Here's how the part is built. I have some questions about the finished solid (model axes, mm). Coordinates: 2 decimals unless noted, no trailing zeros. Loops run counter-clockwise (first coordinate to the right, second up) from the corner with the lowest first, then second, coordinate; pieces in that order, holes last. Notation, with made-up numbers: (-14, -27) -> (23, -27) arc R19 cw to (23, 5) -> close; hole circle Ø8 at (14, -26). An arc over 180 degrees is marked (long way). Answer as a JSON object with one key per item and string values. Group by question number.
1) I'm going to push flat-ended pins straight in: pin 1 (4.5 mm diameter, centred on x = 38.1, y = 88.9, fed in from +Z); pin 2 (1.6 mm diameter, centred on y = 47, z = 2, fed in from +X). Where does each tip first touch, or does it pass through?
2) I need wall thicknesses on probe 1 along Y at (x, z) = (38.1, 1.5); probe 2 along Y at (x, z) = (63.5, 1.9); probe 3 along Y at (x, z) = (40, 0.25). Which ranges of each line are inside material? Lowest first, please. Write a range as [from, to].
3) I want a section at D-D (x = 12.7). Write out the boundary of the cut face in (y, z) (3 decimals).
4) I want a section at B-B (y = 101.6). Write out the boundary of the cut face in (x, z) (3 decimals).
5) I want a section at A-A (x = 63.5). Write out the boundary of the cut face in (y, z) (3 decimals).
6) I want a section at C-C (z = 0.9). Count the separate pieces of the cut face and the enclosed holes in it, then the cut area to 3 significant figures.
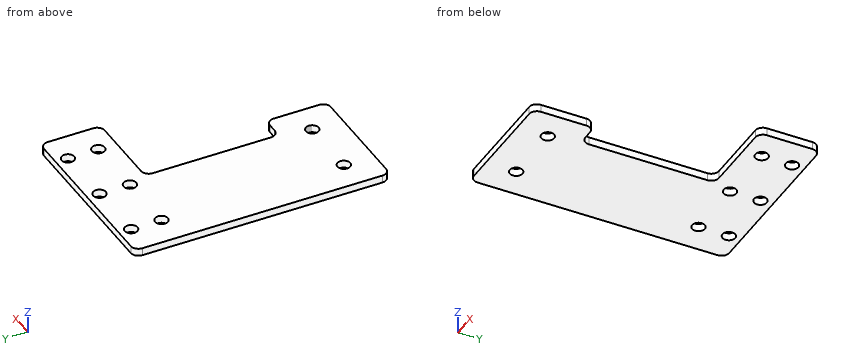
```python
from build123d import *

# Parameters (mm, degrees)
SKETCH1_R           = 2.667
BOSS_EXTRUDE1_DEPTH = 3.175
FILLET1_R           = 3.175


with BuildPart() as part:
    # Sketch1 → Boss-Extrude1 (new body)
    # profile 1 of 2: a face of its own
    with BuildSketch(Plane.XY):
        with BuildLine():
            Line((0, 106.68), (0, 0))
            Line((0, 0), (40.64, 0))
            Line((40.64, 0), (40.64, 11.886803222))
            ThreePointArc((40.64, 11.886803222), (35.433, 12.7), (40.64, 13.513196778))
            Line((40.64, 13.513196778), (40.64, 25.4))
            Line((40.64, 25.4), (40.64, 81.28))
            Line((40.64, 81.28), (50.8, 81.28))
            Line((50.8, 81.28), (76.2, 81.28))
            Line((76.2, 81.28), (76.2, 106.68))
            Line((76.2, 106.68), (0, 106.68))
        make_face()
        with Locations((12.7, 12.7)):
            Circle(SKETCH1_R, mode=Mode.SUBTRACT)
        with Locations((12.7, 88.9)):
            Circle(SKETCH1_R, mode=Mode.SUBTRACT)
        with Locations((12.7, 101.6)):
            Circle(SKETCH1_R, mode=Mode.SUBTRACT)
        with Locations((38.1, 101.6)):
            Circle(SKETCH1_R, mode=Mode.SUBTRACT)
        with Locations((38.1, 88.9)):
            Circle(SKETCH1_R, mode=Mode.SUBTRACT)
        with Locations((63.5, 88.9)):
            Circle(SKETCH1_R, mode=Mode.SUBTRACT)
        with Locations((63.5, 101.6)):
            Circle(SKETCH1_R, mode=Mode.SUBTRACT)
    # profile 2 of 2: a face of its own
    with BuildSketch(Plane.XY):
        with BuildLine():
            Line((40.64, 11.886803222), (40.64, 0))
            Line((40.64, 0), (50.8, 0))
            Line((50.8, 0), (50.8, 25.4))
            Line((50.8, 25.4), (40.64, 25.4))
            Line((40.64, 25.4), (40.64, 13.513196778))
            ThreePointArc((40.64, 13.513196778), (40.735058728, 13.111527034), (40.767, 12.7))
            ThreePointArc((40.767, 12.7), (40.735058728, 12.288472966), (40.64, 11.886803222))
        make_face()
    extrude(amount=BOSS_EXTRUDE1_DEPTH)

    # Fillet1
    fillet1_edges = [part.edges().sort_by_distance(p)[0] for p in [
        (50.8, 25.4, 1.5875),
        (50.8, 0, 1.5875),
        (0, 0, 1.5875),
        (0, 106.68, 1.5875),
        (76.2, 106.68, 1.5875),
        (76.2, 81.28, 1.5875),
        (40.64, 81.28, 1.5875),
        (40.64, 25.4, 1.5875),
    ]]
    fillet(fillet1_edges, radius=FILLET1_R)


solid = part.part
```
Determined:
{
 "1": {"pin 1": "through", "pin 2": "x = 40.64"},
 "2": {"probe 1": "[0, 10.03], [15.37, 86.23], [91.57, 98.93], [104.27, 106.68]", "probe 2": "[81.28, 86.23], [91.57, 98.93], [104.27, 106.68]", "probe 3": "[0, 10.83], [14.57, 87.03], [90.77, 99.73], [103.47, 106.68]"},
 "3": {"outline": "(0, 0) -> (10.033, 0) -> (10.033, 3.175) -> (0, 3.175) -> close; (15.367, 0) -> (86.233, 0) -> (86.233, 3.175) -> (15.367, 3.175) -> close; (91.567, 0) -> (98.933, 0) -> (98.933, 3.175) -> (91.567, 3.175) -> close; (104.267, 0) -> (106.68, 0) -> (106.68, 3.175) -> (104.267, 3.175) -> close"},
 "4": {"outline": "(0, 0) -> (10.033, 0) -> (10.033, 3.175) -> (0, 3.175) -> close; (15.367, 0) -> (35.433, 0) -> (35.433, 3.175) -> (15.367, 3.175) -> close; (40.767, 0) -> (60.833, 0) -> (60.833, 3.175) -> (40.767, 3.175) -> close; (66.167, 0) -> (76.2, 0) -> (76.2, 3.175) -> (66.167, 3.175) -> close"},
 "5": {"outline": "(81.28, 0) -> (86.233, 0) -> (86.233, 3.175) -> (81.28, 3.175) -> close; (91.567, 0) -> (98.933, 0) -> (98.933, 3.175) -> (91.567, 3.175) -> close; (104.267, 0) -> (106.68, 0) -> (106.68, 3.175) -> (104.267, 3.175) -> close"},
 "6": {"separate pieces": "1", "enclosed holes": "8", "area": "5,310 mm^2"}
}
